Can you work these out from the model? Positions are in its coordinate system, mm. Face numbers are marked on the shaded views. Coordinates: 2 decimals unless noted, no trailing zeros. Write each loop counter-clockwise with the first axis right and the second up, starting at its lowest first coordinate (ties: lowest second). Pieces come first, ordered by that corner, then holes. Notation, with made-up numbers: (-24, 32.25) - (1, 32.25) arc R10 cw to (1, 49.25) - close; hole circle Ø11 at (47.25, -27). An arc over 180 degrees is marked (long way). Use one line per item in the form item = value. Start each with the question number.
(1) For pin 1 Ø4 at (x, z) = (-22.5, 17) entering from -Y; pin 2 Ø6 at (x, y) = (-2, 0.5) entering from +Z (3 decimals); pin 3 Ø6 at (x, z) = (-18.5, 10) entering from -Y; pin 4 Ø8 at (x, y) = (-14, -7) entering from +Z, each with a flat end and sliding along its axis, tell me the tip position at first contact or that it passes through.
(2) If we section it at A-A on y = 0: Please give me the cut outline in (x, z).
(3) If we section it at C-C on y = 6.25: Please give me the cut outline in (x, z).
(4) Thinking about a two-plate mould opening in X: for the marked faces 1, 2, 3 and 4, which applies, pulls with the +X half, pulls with the -X half, needs draft (parallel to the pull), parting line crosses it, or undercut?
(5) If we section it at B-B on x = 0: Please give me the cut outline in (y, z), then the cut area to 3 significant figures.
(6) If I drill on probe 1 along Y at (x, z) = (0, 3.35); probe 2 along Z at (x, y) = (-7, -8.5); probe 3 along X at (y, z) = (-0.5, 2.25), over which ranges is the centre line in solid material (lowest first)? Write a range as from..to.
(7) If we section it at D-D on z = 11: Please give me the cut outline in (x, y), then the cut area to 3 significant figures.
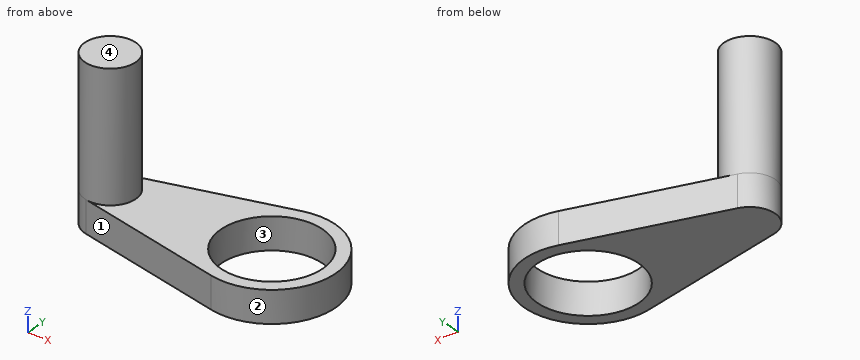
```python
from build123d import *

# Parameters (mm, degrees)
SKETCH_R     = 8
PAD_DEPTH    = 5
SKETCH001_R  = 4
PAD001_DEPTH = 20


with BuildPart() as part:
    # Sketch → Pad (new body)
    with BuildSketch(Plane.XY):
        with BuildLine():
            ThreePointArc((-2.4, -9.7077288796), (10, 0), (-2.4, 9.7077288796))
            Line((-25.96, 3.8830915518), (-2.4, 9.7077288796))
            ThreePointArc((-25.96, 3.8830915518), (-29, 0), (-25.96, -3.8830915518))
            Line((-2.4, -9.7077288796), (-25.96, -3.8830915518))
        make_face()
        Circle(SKETCH_R, mode=Mode.SUBTRACT)
    extrude(amount=PAD_DEPTH)

    # Sketch001 (on Face7 of Pad) → Pad001 (join)
    with BuildSketch(Plane.XY.offset(5)):
        with Locations((-25, 0)):
            Circle(SKETCH001_R)
    extrude(amount=PAD001_DEPTH)


solid = part.part
```
Reported:
q1.pin_1 = -3.97
q1.pin_2 = through
q1.pin_3 = -1.94
q1.pin_4 = 5
q2.outline = (-29, 0) - (-8, 0) - (-8, 5) - (-21, 5) - (-21, 25) - (-29, 25) - close; (8, 0) - (10, 0) - (10, 5) - (8, 5) - close
q3.outline = (-16.39, 0) - (-4.99, 0) - (-4.99, 5) - (-16.39, 5) - close; (4.99, 0) - (7.81, 0) - (7.81, 5) - (4.99, 5) - close
q4.face_1 = pulls with the -X half
q4.face_2 = parting line crosses it
q4.face_3 = undercut
q4.face_4 = needs draft
q5.outline = (-10, 0) - (-8, 0) - (-8, 5) - (-10, 5) - close; (8, 0) - (10, 0) - (10, 5) - (8, 5) - close
q5.area = 20.0 mm2
q6.probe_1 = -10..-8, 8..10
q6.probe_2 = 0..5
q6.probe_3 = -28.97..-7.98, 7.98..9.99
q7.outline = circle Ø8 at (-25, 0)
q7.area = 50.3 mm2
